Verification items for this drawing (mm, ordinates from the low corner). Coordinates: 2 decimals unless noted, no trailing zeros. Write each loop counter-clockwise with the first axis right and the second up, starting at its lowest first coordinate (ties: lowest second). Pieces come first, ordered by that corner, then holes.
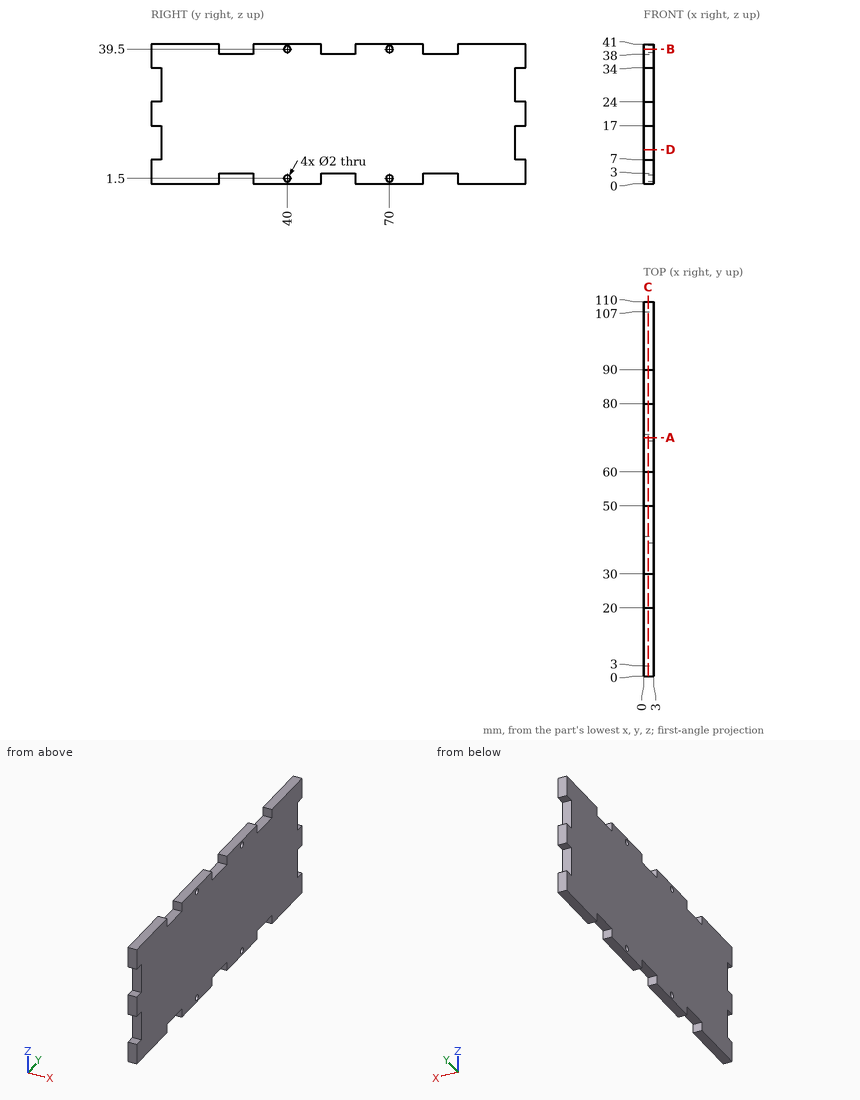
1. Sectioned sample at C-C, the plane x = 1.3. Give the number of separate pieces and of enclosed holes in the cut face, and give its area (3 significant figures).
Computed values:
separate pieces: 1
enclosed holes: 4
area: 4,200 mm2
2. Sectioned sample at B-B, the plane z = 39.5. Record the boundary of the cut face in (x, y), and give its area (3 significant figures).
Computed values:
outline: (0, 0) - (3, 0) - (3, 20) - (0, 20) - close; (0, 30) - (3, 30) - (3, 39) - (0, 39) - close; (0, 41) - (3, 41) - (3, 50) - (0, 50) - close; (0, 60) - (3, 60) - (3, 69) - (0, 69) - close; (0, 71) - (3, 71) - (3, 80) - (0, 80) - close; (0, 90) - (3, 90) - (3, 110) - (0, 110) - close
area: 228 mm2
3. Gauge pin test, flat ends, axial feed: pin 1 Ø10 at (y, z) = (63, 18.5) entering from -X; pin 2 Ø1.5 at (x, y) = (1, 24.5) entering from -Z; pin 3 Ø1.5 at (x, y) = (2, 85) entering from +Z. Record the tip position at first contact, or that the pin passes through.
Computed values:
pin 1: stops at x = 0
pin 2: stops at z = 3
pin 3: stops at z = 38
4. Sectioned sample at D-D, the plane z = 10. Record the boundary of the cut face in (x, y).
Computed values:
outline: (0, 3) - (3, 3) - (3, 107) - (0, 107) - close
5. Sectioned sample at A-A, the plane y = 70. Record the boundary of the cut face in (x, z).
Computed values:
outline: (0, 0) - (3, 0) - (3, 0.5) - (0, 0.5) - close; (0, 2.5) - (3, 2.5) - (3, 38.5) - (0, 38.5) - close; (0, 40.5) - (3, 40.5) - (3, 41) - (0, 41) - close
6. Thickness scan on line 1 along Z through (x, y) = (1.65, 40); line 2 along Z through (x, y) = (1.1, 55.5); line 3 along Y through (x, z) = (2.15, 16.5). Record the ranges inside material, lowest first.
Computed values:
line 1: z = 0 to 0.5, 2.5 to 38.5, 40.5 to 41
line 2: z = 3 to 38
line 3: y = 3 to 107
